```python
from build123d import *

# Parameters (mm, degrees)
BOSS_EXTRUDE1_DEPTH = 204


with BuildPart() as part:
    # Szkic1 → Boss-Extrude1 (new body)
    with BuildSketch(Plane.XY):
        with BuildLine():
            Line((92.010000436, 51.077414838), (101.009999564, 51.077414838))
            Line((101.009999564, 51.077414838), (101.009999564, 50.859999228))
            ThreePointArc((101.009999564, 50.859999228), (100.95142109, 50.718578281), (100.810000144, 50.659999808))
            Line((100.810000144, 50.659999808), (100.710000374, 50.659999808))
            ThreePointArc((100.710000374, 50.659999808), (100.568578753, 50.601421054), (100.51, 50.459999434))
            Line((100.51, 50.459999434), (100.51, 48.459999434))
            ThreePointArc((100.51, 48.459999434), (100.623168266, 48.085202764), (100.943422808, 47.859999237))
            ThreePointArc((100.943422808, 47.859999237), (101.030642298, 47.766174714), (100.936817775, 47.678955223))
            Line((100.936817775, 47.678955223), (100.57727329, 47.678955223))
            ThreePointArc((100.57727329, 47.678955223), (100.041576562, 47.900848073), (99.819683712, 48.436544801))
            Line((99.819683712, 48.436544801), (99.819683712, 49.359999626))
            ThreePointArc((99.819683712, 49.359999626), (99.743947721, 49.542842483), (99.561104865, 49.618578474))
            Line((99.561104865, 49.618578474), (93.458895135, 49.618578474))
            ThreePointArc((93.458895135, 49.618578474), (93.276052279, 49.542842483), (93.200316288, 49.359999626))
            Line((93.200316288, 49.359999626), (93.200316288, 48.436544801))
            ThreePointArc((93.200316288, 48.436544801), (92.978423438, 47.900848073), (92.44272671, 47.678955223))
            Line((92.44272671, 47.678955223), (92.083182225, 47.678955223))
            ThreePointArc((92.083182225, 47.678955223), (91.989357702, 47.766174714), (92.076577192, 47.859999237))
            ThreePointArc((92.076577192, 47.859999237), (92.396831734, 48.085202764), (92.51, 48.459999434))
            Line((92.51, 48.459999434), (92.51, 50.459999434))
            ThreePointArc((92.51, 50.459999434), (92.451421247, 50.601421054), (92.309999626, 50.659999808))
            Line((92.309999626, 50.659999808), (92.209999856, 50.659999808))
            ThreePointArc((92.209999856, 50.659999808), (92.06857891, 50.718578281), (92.010000436, 50.859999228))
            Line((92.010000436, 50.859999228), (92.010000436, 51.077414838))
        make_face()
    extrude(amount=BOSS_EXTRUDE1_DEPTH)


solid = part.part
```
Source: CAD feature listing. Evaluate the final solid. Frame: model axes, mm. Round coordinates to 2 decimals unless told otherwise and drop trailing zeros. Write each loop counter-clockwise with the first axis right and the second up, starting at its lowest first coordinate (ties: lowest second). Pieces come first, ordered by that corner, then holes. Notation, with made-up numbers: M 26,59 L 58,59 A27 cw 58,96 Z; hole C 8,-36 d6. An arc over 180 degrees is marked long. Use CSV: the item, a comma, the result in double quotes. Start each with the question number.
Q1. Pull-direction query (X, two-part tool) for faces 1 (the face through (97, 49.619, 101)), 2 (the face through (96, 50, 204)); classes: +X half, -X half, draft (parallel to the pull), parting line (faces both ways), or undercut.
Q2. Cut plane A-A on z = 153. Output: boundary loops of the cut face in (x, y).
Q3. Line query: line 1 (X direction, y = 49.25, z = 123); line 2 (Y direction, x = 96.5, z = 167.5); line 3 (X direction, y = 47.8, z = 180.5). Output: solid intervals per line, ascending. Write a range as from..to.
Q4. First-contact query: P1, Ø1, axis at y = 50, z = 144, coming from the -X side; P2, Ø1.8, axis at x = 95.5, z = 99.5, coming from the -Y side; P3, Ø0.7, axis at y = 48.5, z = 112.5, coming from the +X side. Flat tips, straight axial feed; report the tip coordinate or a pass-through.
Q5. Cut plane B-B on x = 95.25. Output: boundary loops of the cut face in (y, z).
Results found:
1,face 1,"undercut"
1,face 2,"draft"
2,outline,"M 92.01,50.86 A0.2 ccw 92.21,50.66 L 92.31,50.66 A0.2 cw 92.51,50.46 L 92.51,48.46 A0.6 cw 92.08,47.86 A0.09 ccw 92.08,47.68 L 92.44,47.68 A0.76 ccw 93.2,48.44 L 93.2,49.36 A0.26 cw 93.46,49.62 L 99.56,49.62 A0.26 cw 99.82,49.36 L 99.82,48.44 A0.76 ccw 100.58,47.68 L 100.94,47.68 A0.09 ccw 100.94,47.86 A0.6 cw 100.51,48.46 L 100.51,50.46 A0.2 cw 100.71,50.66 L 100.81,50.66 A0.2 ccw 101.01,50.86 L 101.01,51.08 L 92.01,51.08 Z"
3,line 1,"92.51..93.2, 99.82..100.51"
3,line 2,"49.62..51.08"
3,line 3,"91.99..92.85, 100.17..101.03"
4,P1,"x = 92.51"
4,P2,"y = 49.62"
4,P3,"x = 100.58"
5,outline,"M 49.62,0 L 51.08,0 L 51.08,204 L 49.62,204 Z"
